Could you check a few things on this model? Use its own coordinates, in mm. Face numbers are marked on the shaded views. A direction names the side the tool comes from. Coordinates: 2 decimals unless noted, no trailing zeros. Write each loop counter-clockwise with the first axis right and the second up, starting at its lowest first coordinate (ties: lowest second). Pieces come first, ordered by that corner, then holes. Notation, with made-up numbers: M -10.5,67.25 L 20.5,67.25 A36 cw 20.5,105.25 Z; hole C 35,77.25 d11. An arc over 180 degrees is marked long. Write item = value, one per line.
Autodesk Inventor part; units mm, degrees
ref_plane "РабПлоскость1" through (0.4806, 50.2, -0.1709) normal (-1, 0, 0) x (0, -1, 0)
ref_plane "YZ Plane" through (0, 0, 0) normal (1, 0, 0) x (0, 1, 0)
ref_plane "XZ Plane" through (0, 0, 0) normal (0, 1, 0) x (-1, 0, 0)
sketch "Эскиз1" plane through (0, 0, 0) normal (0, 1, 0) x (-1, 0, 0)
  arc A0 (4.0194, -3.1709) -> (-7.7806, -3.1709) centre (-1.8806, -45.2594) ccw
  line L0 (-7.7806, -3.1709) -> (-7.7806, 2.8291)
  line L1 (-7.7806, 2.8291) -> (4.0194, 2.8291)
  line L2 (4.0194, 2.8291) -> (4.0194, -3.1709)
  point P0 (0, -39)
  dimension "d1" = 6
  dimension "d12" = 11.8
extrude "Выдавливание1" add sketch "Эскиз1" along normal blind 50.2
sketch "Эскиз2" plane through (0, 50.2, 0) normal (0, 1, 0) x (1, 0, 0)
  line L0 (-4.0194, -2.8291) -> (7.7806, -2.8291)
  line L1 (1.8806, -2.8291) -> (1.8806, 0.1709)
  circle A0 centre (1.8806, 0.1709) radius 1.4
  point P0 (0, 0)
  dimension "d5" = 3
  dimension "d6" = 2.8
extrude "Выдавливание2" cut sketch "Эскиз2" against normal blind 10
sketch "Эскиз3" plane through (0, 0, 0) normal (0, -1, 0) x (1, 0, 0)
  line L0 (-4.0194, 2.8291) -> (7.7806, 2.8291)
  line L1 (1.8806, 2.8291) -> (1.8806, -0.1709)
  circle A0 centre (1.8806, -0.1709) radius 1.4
  point P0 (0, 0)
  dimension "d9" = 3
extrude "Выдавливание3" cut sketch "Эскиз3" against normal blind 10
sketch "Эскиз4" plane through (0, 0, 0) normal (0, -1, 0) x (1, 0, 0)
  arc A0 (7.7806, -3.1709) -> (-4.0194, -3.1709) centre (1.8806, -45.2594) ccw
  line L0 (1.8806, -2.7594) -> (-4.0194, -2.7594)
  line L1 (-4.0194, -3.1709) -> (-4.0194, 2.8291)
  line L2 (-4.0194, 2.8291) -> (-19.0194, 2.8291)
  line L3 (-19.0194, 2.8291) -> (-19.0194, -2.7594)
  line L4 (-19.0194, -2.7594) -> (-4.0194, -2.7594)
  line L5 (-4.0194, -2.7594) -> (-4.0194, 2.8291)
  line L6 (7.7806, 2.8291) -> (7.7806, -3.1709)
  line L7 (7.7806, 2.8291) -> (22.7806, 2.8291)
  line L8 (22.7806, 2.8291) -> (22.7806, -2.7594)
  line L9 (22.7806, -2.7594) -> (7.7806, -2.7594)
  line L10 (7.7806, -2.7594) -> (7.7806, 2.8291)
  point P0 (0, 0)
  dimension "d13" = 15
  dimension "d16" = 15
extrude "Выдавливание4" add sketch "Эскиз4" against normal up to surface (50.2 mm away) contours L4 L3 L2 L1 | L6 L7 L8 L9
ref_plane "РабПлоскость1" through (0.4806, 50.2, -0.1709) normal (-1, 0, 0) x (0, -1, 0)
properties part number "joint3_rot_con" material "Пластик АБС"
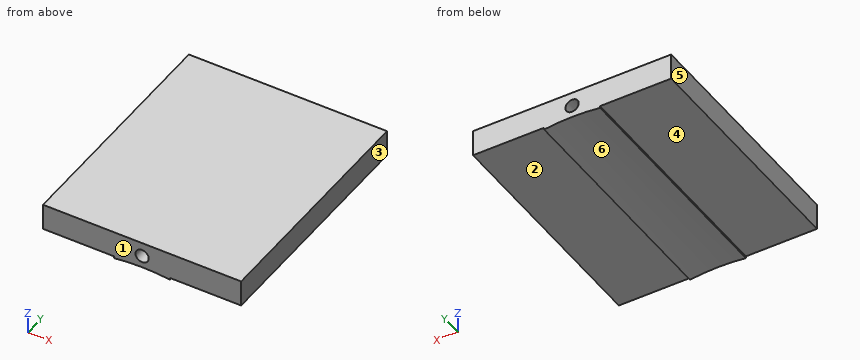
Item 1: Imagine slicing it at C-C (y = 44). Write out the boundary of the cut face in (x, z).
Numbers:
outline = M -19.02,-2.76 L -4.02,-2.76 L -4.02,-3.17 A42.5 cw 7.78,-3.17 L 7.78,-2.76 L 22.78,-2.76 L 22.78,2.83 L -19.02,2.83 Z; hole C 1.88,-0.17 d2.8
Item 2: For the marked faces 1 and 2, which set-ups out of +Z, -Z, +X, -X, +Y, -Y let a thin tool reach every point of the face, with its end or its side?
Numbers:
face_1 = +Z, -Z, +X, -X, -Y
face_2 = -Z, +X, +Y, -Y
Item 3: Imagine slicing it at B-B (z = -1). Write out the boundary of the cut face in (x, y).
Numbers:
outline = M -19.02,0 L 0.75,0 L 0.75,10 L 3.01,10 L 3.01,0 L 22.78,0 L 22.78,50.2 L 3.01,50.2 L 3.01,40.2 L 0.75,40.2 L 0.75,50.2 L -19.02,50.2 Z
Item 4: Imagine slicing it at A-A (y = 23). Write out the boundary of the cut face in (x, z), and give its area (3 significant figures).
Numbers:
outline = M -19.02,-2.76 L -4.02,-2.76 L -4.02,-3.17 A42.5 cw 7.78,-3.17 L 7.78,-2.76 L 22.78,-2.76 L 22.78,2.83 L -19.02,2.83 Z
area = 235 mm²
Item 5: If we mould it in two halves opening along X, with no side actions, what happens to the marked faces 3, 4, 5 and 6? For each: pulls with the +X half, pulls with the -X half, needs draft (parallel to the pull), parting line crosses it, or undercut.
Numbers:
face_3 = pulls with the +X half
face_4 = needs draft
face_5 = pulls with the -X half
face_6 = undercut
Item 6: If I drill on line 1 along Z through (x, y) = (-9, 34); line 2 along X through (y, z) = (6.5, -0.75); line 3 along X through (y, z) = (41, -0.9), over which ranges is the centre line in solid material (lowest first)?
Numbers:
line_1 = -2.76 to 2.83
line_2 = -19.02 to 0.61, 3.16 to 22.78
line_3 = -19.02 to 0.69, 3.08 to 22.78
Item 7: I'm going to push flat-ended pins straight in: P1, Ø2.5, axis at x = 1.88, z = -0.17, coming from the +Y side; P2, Ø2, axis at x = 1.88, z = -0.17, coming from the -Y side; P3, Ø12, axis at x = -12.5, y = 15.5, coming from the -Z side. Where does each tip first touch, or does it pass through?
Numbers:
P1 = 40.2
P2 = 10
P3 = -2.76
Item 8: Imagine slicing it at D-D (x = -11). Write out the boundary of the cut face in (y, z).
Numbers:
outline = M 0,-2.76 L 50.2,-2.76 L 50.2,2.83 L 0,2.83 Z
